Verification items for this drawing (mm, ordinates from the low corner). A direction names the side the tool comes from. Round coordinates to 2 decimals unless told otherwise and drop trailing zeros. Write each loop counter-clockwise with the first axis right and the second up, starting at its lowest first coordinate (ties: lowest second). Pieces come first, ordered by that corner, then holes. Notation, with made-up numbers: M 56.25,-7 L 60.25,-7 A31 ccw 60.25,23 Z; hole C 84.25,-18 d3. An arc over 180 degrees is marked long. Write each question's results on one line, items separated by ' | '.
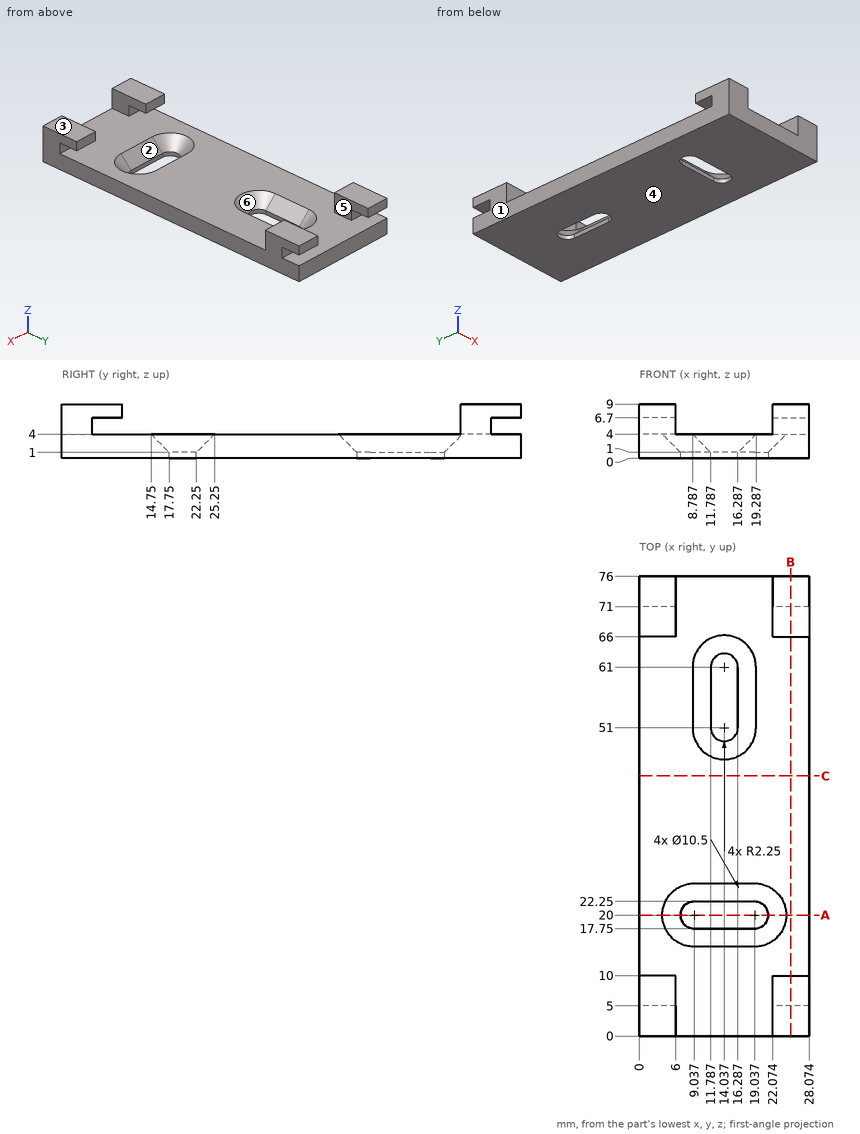
1) Sectioned sample at A-A, the plane y = 20. Record the cut outline in (x, z).
Calculated:
outline: M 0,0 L 6.79,0 L 6.79,1 L 3.79,4 L 0,4 Z; M 21.29,0 L 28.07,0 L 28.07,4 L 24.29,4 L 21.29,1 Z
2) Draft check along X on the marked faces 1, 2 and 3. Enter one of: pulls with the +X half, pulls with the -X half, needs draft (parallel to the pull), parting line crosses it, or undercut.
Calculated:
face 1: pulls with the -X half | face 2: undercut | face 3: needs draft
3) Sectioned sample at C-C, the plane y = 43. Record the cut outline in (x, z).
Calculated:
outline: M 0,0 L 28.07,0 L 28.07,4 L 0,4 Z
4) Depth check by flat-ended pin: P1, Ø1.4, axis at x = 26.5, z = 5.5, coming from the +Y side; P2, Ø10, axis at x = 12.5, y = 52, coming from the +Z side. Enter the tip coordinate at first touch or a pass-through.
Calculated:
P1: stops at y = 71 | P2: stops at z = 4
5) Sectioned sample at B-B, the plane x = 25. Record the cut outline in (y, z).
Calculated:
outline: M 0,0 L 76,0 L 76,4 L 71,4 L 71,6.7 L 76,6.7 L 76,9 L 66,9 L 66,4 L 5,4 L 5,6.7 L 10,6.7 L 10,9 L 0,9 Z
6) Access from +Z, -Z, +X, -X, +Y, -Y to the whole of each face (thin tool, end or side, straight path). Record for the marked faces 4, 5 and 6.
Calculated:
face 4: -Z, +X, -X, +Y, -Y | face 5: +Z, +Y, -Y | face 6: +Z
7) Material ranges on line 1 (Y direction, x = 26.25, z = 4.75); line 2 (Z direction, x = 26.75, y = 7); line 3 (Z direction, x = 11.5, y = 35), recorded low to high. Write a range as [from, to].
Calculated:
line 1: y = [0, 5], [66, 71] | line 2: z = [0, 4], [6.7, 9] | line 3: z = [0, 4]
